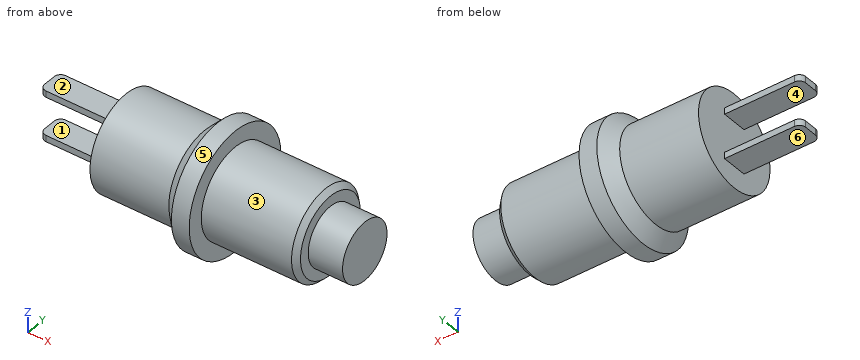
Autodesk Inventor part; units mm, degrees
ref_plane "YZ Plane" through (0, 0, 0) normal (1, 0, 0) x (0, 1, 0)
ref_plane "XZ Plane" through (0, 0, 0) normal (0, 1, 0) x (-1, 0, 0)
ref_plane "XY Plane" through (0, 0, 0) normal (0, 0, 1) x (1, 0, 0)
sketch "Esquisse1" plane through (0, 0, 0) normal (0, 0, 1) x (1, 0, 0)
  line L0 (-14.8768, 0) -> (-3.0909, 0)
  line L1 (0, 3.7) -> (0, 0)
  line L2 (8.6, 4.75) -> (7.2, 4.75)
  line L3 (8.6, 3.5) -> (8.6, 4.75)
  line L4 (8.6, 3.5) -> (16.1, 3.5)
  line L5 (16.1, 3.5) -> (16.1, 2.3)
  line L6 (16.1, 2.3) -> (18.8, 2.3)
  line L7 (18.8, 2.3) -> (18.8, 3)
  line L8 (0, 3.7) -> (6.2, 3.7)
  line L9 (6.2, 3.7) -> (7.2, 4.75)
  line L10 (18.8, 2.3) -> (18.8, 0)
  line L11 (18.8, 0) -> (0, 0)
  dimension "d4" = 9.5
  dimension "d5" = 7
  dimension "d6" = 4.6
  dimension "d9" = 1.4
  dimension "d10" = 7.4
  dimension "d11" = 1
  dimension "d12" = 7.5
  dimension "d15" = 2.7
  dimension "d16" = 18.8
revolve "Révolution1" add sketch "Esquisse1" angle 360 about axis through (-14.8768, 0, 0) along (1, 0, 0)
thread "Filetage1"
chamfer "Chanfrein1" distance 0.4 angle 45 1 edges at (16.1, -3.5, 0)
sketch "Esquisse2" plane through (0, 0, 0) normal (-1, 0, 0) x (0, 0, 1)
  line L0 (2, -1) -> (1.5, -1)
  line L1 (1.5, -1) -> (1.5, 1)
  line L2 (1.5, 1) -> (2, 1)
  line L3 (2, 1) -> (2, -1)
  line L4 (-1.5, -1) -> (-2, -1)
  line L5 (-2, -1) -> (-2, 1)
  line L6 (-2, 1) -> (-1.5, 1)
  line L7 (-1.5, 1) -> (-1.5, -1)
  line L8 (0, -6.65) -> (0, 6.65) construction
  line L9 (-6.65, 0) -> (6.65, 0) construction
  point P0 (0, 0)
  dimension "d23" = 0.5
  dimension "d24" = 2
  dimension "d25" = 3
extrude "Extrusion1" add sketch "Esquisse2" along normal blind 6
fillet "Congé1" radius 0.5 4 edges at (-6, -1, 1.75) (-6, 1, 1.75) (-6, 1, -1.75) (-6, -1, -1.75)
properties part number "Bouton"
Design review of the part built by this model. Coordinates are the model's own, in mm. Face numbers are marked on the shaded views. A direction names the side the tool comes from. Give positions to 0.01 mm unless a question says otherwise; leave off trailing zeros. Order: outer loops, then holes, each group sorted by start corner. A loop starts at its lowest first (then second) coordinate and runs counter-clockwise, first axis right, second up. Notation, with made-up numbers: (-3, -35) -> (33, -35) arc R18 ccw to (33, -19) -> close; hole circle Ø7 at (14, 23.25). An arc over 180 degrees is marked (long way). Write each question's results on one line, items separated by ' | '. Start each with the question number.
Q1. Add section A-A on z = 0. Give the boundary of the cut face in (x, y).
Q2. Mouldability with a two-part tool opening along Z and no side actions: class the marked faces 4, 5 and 6 as +Z half, -Z half, draft (parallel to the pull), parting line (faces both ways), or undercut.
Q3. For pin 1 (1.6 mm diameter, centred on x = -3, y = 0, fed in from +Z); pin 2 (2 mm diameter, centred on y = -1.5, z = -3, fed in from -X); pin 3 (2 mm diameter, centred on x = 9, z = 3.5, fed in from +Y), all flat-tipped, find the tip position at first contact; note any pin that passes through.
Q4. Machinability: for the marked faces 1, 2 and 3, which of the approach directions +Z, -Z, +X, -X, +Y, -Y give a long, thin tool a straight path to every point of the face, cutting with its end or side? Answer none if there is none.
Q5. Add section C-C on x = 9.75. Give the boundary of the cut face in (y, z).
Q6. Wall thickness on L1, parallel to Z at x = -3, y = 0.5; L2, parallel to X at y = -0.5, z = 0.5; L3, parallel to X at y = 2.75, z = -0.75: over which ranges is each line inside the solid? List them lowest first. Write a range as from..to.
Q7. Add section B-B on y = 0. Give the boundary of the cut face in (x, z).
Found:
1) outline: (0, -3.7) -> (6.2, -3.7) -> (7.2, -4.75) -> (8.6, -4.75) -> (8.6, -3.5) -> (15.7, -3.5) -> (16.1, -3.1) -> (16.1, -2.3) -> (18.8, -2.3) -> (18.8, 2.3) -> (16.1, 2.3) -> (16.1, 3.1) -> (15.7, 3.5) -> (8.6, 3.5) -> (8.6, 4.75) -> (7.2, 4.75) -> (6.2, 3.7) -> (0, 3.7) -> close
2) face 4: undercut | face 5: parting line | face 6: -Z half
3) pin 1: stops at z = 2 | pin 2: stops at x = 0 | pin 3: stops at y = 3.99
4) face 1: -X, +Y, -Y | face 2: +Z, -X, +Y, -Y | face 3: +X
5) outline: circle Ø7 at (0, 0)
6) L1: z = -2..-1.5, 1.5..2 | L2: x = 0..18.8 | L3: x = 0..16.1
7) outline: (-6, -2) -> (0, -2) -> (0, -3.7) -> (6.2, -3.7) -> (7.2, -4.75) -> (8.6, -4.75) -> (8.6, -3.5) -> (15.7, -3.5) -> (16.1, -3.1) -> (16.1, -2.3) -> (18.8, -2.3) -> (18.8, 2.3) -> (16.1, 2.3) -> (16.1, 3.1) -> (15.7, 3.5) -> (8.6, 3.5) -> (8.6, 4.75) -> (7.2, 4.75) -> (6.2, 3.7) -> (0, 3.7) -> (0, 2) -> (-6, 2) -> (-6, 1.5) -> (0, 1.5) -> (0, -1.5) -> (-6, -1.5) -> close
